For this review, take the finished solid that the model builds, in its own axes (mm). Face numbers are marked on the shaded views. Round coordinates to 2 decimals unless told otherwise and drop trailing zeros. Order: outer loops, then holes, each group sorted by start corner. A loop starts at its lowest first (then second) coordinate and runs counter-clockwise, first axis right, second up. Notation, with made-up numbers: M -26.5,3 L -17.5,3 A20 ccw -17.5,16 Z; hole C 74.25,8 d10. An arc over 180 degrees is marked long. Use a Markdown table: item, result.
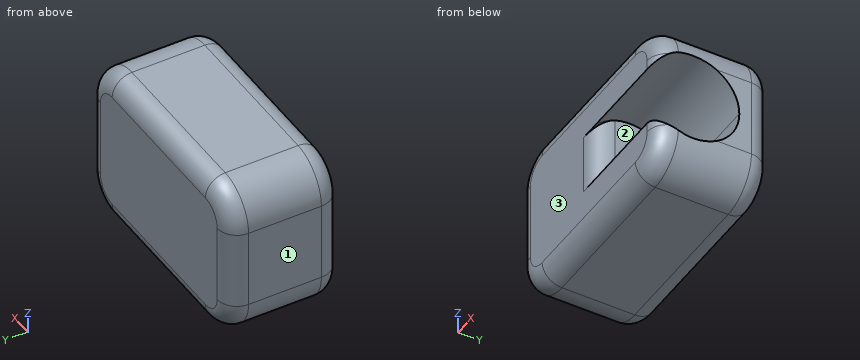
from build123d import *

# Parameters (mm, degrees)
F0_W         = 152.4
F0_H         = 101.6
F1_DEPTH     = 72.136
F3_DEPTH     = 69.088
F4_T1_DEPTH  = 199.136
F5_T1_DEPTH  = 101.6
F5_T3_DEPTH  = 50.8
F5_T5_DEPTH  = 37.8518945456
F5_T7_DEPTH  = 37.8518945456
F5_T12_DEPTH = 102.0962109088
F5_S13_R     = 29.4462721735
F5_T14_DEPTH = 53
F5_T16_ANGLE = 89.9999999994
F5_T18_ANGLE = 89.9999999994
F5_T20_ANGLE = 89.9999999994
F5_T22_ANGLE = 89.9999999994
F5_T24_ANGLE = 89.9999999994
F5_T26_ANGLE = 89.9999999994
F5_T28_ANGLE = 89.9999999994
F5_T30_ANGLE = 89.9999999994


# Not quite as in the source:
# - a fillet or chamfer that OpenCascade refuses, or shapes differently, is made with other operations: its cross-section is extruded or revolved along the edge and cut away or added


with BuildPart() as f1:
    # F0 (on Front) → F1 (new body)
    with BuildSketch(Plane.XZ):
        Rectangle(F0_W, F0_H)
    extrude(amount=F1_DEPTH)

    # F2 (on face) → F3 (cut)
    with BuildSketch(Plane.YZ.offset(76.2)):
        with BuildLine():
            Line((-72.136, -19.2981054544), (-72.136, 19.2981054544))
            ThreePointArc((-72.136, 19.2981054544), (-79.3411824793, 0), (-72.136, -19.2981054544))
        make_face()
        with BuildLine():
            ThreePointArc((-72.136, -19.2981054544), (-39.5952558372, -27.5862295855), (-20.4486381322, 0))
            ThreePointArc((-20.4486381322, 0), (-39.5952558372, 27.5862295855), (-72.136, 19.2981054544))
            Line((-72.136, 19.2981054544), (-72.136, -19.2981054544))
        make_face()
    extrude(amount=-F3_DEPTH, mode=Mode.SUBTRACT)

    # F4: fillet of radius 25.4 on 4 edges, made by hand

    # F4_s2 → F4_t1 (cut)
    with BuildSketch(Plane.XZ.offset(-63.5)):
        with BuildLine():
            ThreePointArc((50.8, -50.8), (68.7605122421, -43.3605122421), (76.2, -25.4))
            Line((76.2, -25.4), (76.2, -50.8))
            Line((76.2, -50.8), (50.8, -50.8))
        make_face()
        with BuildLine():
            ThreePointArc((-50.8, -50.8), (-68.7605122421, -43.3605122421), (-76.2, -25.4))
            Line((-76.2, -25.4), (-76.2, -50.8))
            Line((-76.2, -50.8), (-50.8, -50.8))
        make_face()
        with BuildLine():
            ThreePointArc((76.2, 25.4), (68.7605122421, 43.3605122421), (50.8, 50.8))
            Line((50.8, 50.8), (76.2, 50.8))
            Line((76.2, 50.8), (76.2, 25.4))
        make_face()
        with BuildLine():
            ThreePointArc((-76.2, 25.4), (-68.7605122421, 43.3605122421), (-50.8, 50.8))
            Line((-50.8, 50.8), (-76.2, 50.8))
            Line((-76.2, 50.8), (-76.2, 25.4))
        make_face()
    extrude(amount=F4_T1_DEPTH, mode=Mode.SUBTRACT)

    # F5: fillet of radius 12.7 on 16 edges, made by hand

    # F5_s2 → F5_t1 (cut)
    with BuildSketch(Plane.YZ.offset(-50.8)):
        with BuildLine():
            ThreePointArc((-72.136, 38.1), (-68.4162561211, 47.0802561211), (-59.436, 50.8))
            Line((-59.436, 50.8), (-72.136, 50.8))
            Line((-72.136, 50.8), (-72.136, 38.1))
        make_face()
        with BuildLine():
            ThreePointArc((0, 38.1), (-3.7197438789, 47.0802561211), (-12.7, 50.8))
            Line((-12.7, 50.8), (0, 50.8))
            Line((0, 50.8), (0, 38.1))
        make_face()
        with BuildLine():
            ThreePointArc((-12.7, -50.8), (-3.7197438789, -47.0802561211), (0, -38.1))
            Line((0, -38.1), (0, -50.8))
            Line((0, -50.8), (-12.7, -50.8))
        make_face()
        with BuildLine():
            ThreePointArc((-59.436, -50.8), (-68.4162561211, -47.0802561211), (-72.136, -38.1))
            Line((-72.136, -38.1), (-72.136, -50.8))
            Line((-72.136, -50.8), (-59.436, -50.8))
        make_face()
    extrude(amount=F5_T1_DEPTH, mode=Mode.SUBTRACT)

    # F5_s4 → F5_t3 (cut)
    with BuildSketch(Plane.XY.offset(-25.4)):
        with BuildLine():
            ThreePointArc((-63.5, 0), (-72.4802561211, -3.7197438789), (-76.2, -12.7))
            Line((-76.2, -12.7), (-76.2, 0))
            Line((-76.2, 0), (-63.5, 0))
        make_face()
        with BuildLine():
            ThreePointArc((63.5, 0), (72.4802561211, -3.7197438789), (76.2, -12.7))
            Line((76.2, -12.7), (76.2, 0))
            Line((76.2, 0), (63.5, 0))
        make_face()
        with BuildLine():
            ThreePointArc((-63.5, -72.136), (-72.4802561211, -68.4162561211), (-76.2, -59.436))
            Line((-76.2, -59.436), (-76.2, -72.136))
            Line((-76.2, -72.136), (-63.5, -72.136))
        make_face()
    extrude(amount=F5_T3_DEPTH, mode=Mode.SUBTRACT)

    # F5_s6 → F5_t5 (cut)
    with BuildSketch(Plane.XY.offset(-12.4518945456)):
        with BuildLine():
            ThreePointArc((63.5, -72.136), (72.4802561211, -68.4162561211), (76.2, -59.436))
            Line((76.2, -59.436), (76.2, -72.136))
            Line((76.2, -72.136), (63.5, -72.136))
        make_face()
    extrude(amount=F5_T5_DEPTH, mode=Mode.SUBTRACT)

    # F5_s8 → F5_t7 (cut)
    with BuildSketch(Plane.XY.offset(-25.4)):
        with BuildLine():
            ThreePointArc((63.5, -72.136), (72.4802561211, -68.4162561211), (76.2, -59.436))
            Line((76.2, -59.436), (76.2, -72.136))
            Line((76.2, -72.136), (63.5, -72.136))
        make_face()
    extrude(amount=F5_T7_DEPTH, mode=Mode.SUBTRACT)


with BuildPart() as f5_tool10:
    # F5_s11 → F5_t12 (new body)
    with BuildSketch(Plane.XY.offset(-51.0481054544)):
        with BuildLine():
            ThreePointArc((-5.588, -72.136), (3.3922561211, -68.4162561211), (7.112, -59.436))
            Line((7.112, -59.436), (7.112, -72.136))
            Line((7.112, -72.136), (-5.588, -72.136))
        make_face()
    extrude(amount=F5_T12_DEPTH)

    # F5_s13 → F5_t14 (intersect, symmetric)
    with BuildSketch(Plane.YZ.offset(0.8)):
        with Locations((-49.8949103057, 0)):
            Circle(F5_S13_R)
    extrude(amount=F5_T14_DEPTH, both=True, mode=Mode.INTERSECT)


with BuildPart() as f1_1:
    add(f1.part)

    # F5_t9: cut F5_tool10
    add(f5_tool10.part, mode=Mode.SUBTRACT)

    # F5_s15 → F5_t16 (revolve, cut)
    with BuildSketch(Plane.YZ.offset(-50.7999999999)):
        with BuildLine():
            ThreePointArc((0, -38.1), (-3.7197438789, -47.0802561211), (-12.7, -50.8))
            Line((-12.7, -50.8), (0, -50.8))
            Line((0, -50.8), (0, -38.1))
        make_face()
    revolve(axis=Axis((-50.7999999999, 0, -25.3999999999), (0, 1, 0)), revolution_arc=F5_T16_ANGLE, mode=Mode.SUBTRACT)

    # F5_s17 → F5_t18 (revolve, cut)
    with BuildSketch(Plane.XY.offset(25.3999999999)):
        with BuildLine():
            ThreePointArc((-63.5, 0), (-72.4802561211, -3.7197438789), (-76.2, -12.7))
            Line((-76.2, -12.7), (-76.2, 0))
            Line((-76.2, 0), (-63.5, 0))
        make_face()
    revolve(axis=Axis((-50.7999999999, 0, 25.3999999999), (0, 1, 0)), revolution_arc=F5_T18_ANGLE, mode=Mode.SUBTRACT)

    # F5_s19 → F5_t20 (revolve, cut)
    with BuildSketch(Plane.YZ.offset(50.7999999999)):
        with BuildLine():
            ThreePointArc((0, 38.1), (-3.7197438789, 47.0802561211), (-12.7, 50.8))
            Line((-12.7, 50.8), (0, 50.8))
            Line((0, 50.8), (0, 38.1))
        make_face()
    revolve(axis=Axis((50.7999999999, 0, 25.3999999999), (0, 1, 0)), revolution_arc=F5_T20_ANGLE, mode=Mode.SUBTRACT)

    # F5_s21 → F5_t22 (revolve, cut)
    with BuildSketch(Plane.XY.offset(-25.3999999999)):
        with BuildLine():
            ThreePointArc((63.5, 0), (72.4802561211, -3.7197438789), (76.2, -12.7))
            Line((76.2, -12.7), (76.2, 0))
            Line((76.2, 0), (63.5, 0))
        make_face()
    revolve(axis=Axis((50.7999999999, 0, -25.3999999999), (0, 1, 0)), revolution_arc=F5_T22_ANGLE, mode=Mode.SUBTRACT)

    # F5_s23 → F5_t24 (revolve, cut)
    with BuildSketch(Plane.XY.offset(-25.3999999999)):
        with BuildLine():
            ThreePointArc((76.2, -59.436), (72.4802561211, -68.4162561211), (63.5, -72.136))
            Line((63.5, -72.136), (76.2, -72.136))
            Line((76.2, -72.136), (76.2, -59.436))
        make_face()
    revolve(axis=Axis((50.7999999999, -72.136, -25.3999999999), (0, 1, 0)), revolution_arc=F5_T24_ANGLE, mode=Mode.SUBTRACT)

    # F5_s25 → F5_t26 (revolve, cut)
    with BuildSketch(Plane.XY.offset(25.3999999999)):
        with BuildLine():
            ThreePointArc((-63.5, -72.136), (-72.4802561211, -68.4162561211), (-76.2, -59.436))
            Line((-76.2, -59.436), (-76.2, -72.136))
            Line((-76.2, -72.136), (-63.5, -72.136))
        make_face()
    revolve(axis=Axis((-50.7999999999, -72.136, 25.3999999999), (0, 1, 0)), revolution_arc=F5_T26_ANGLE, mode=Mode.SUBTRACT)

    # F5_s27 → F5_t28 (revolve, cut)
    with BuildSketch(Plane.YZ.offset(50.7999999999)):
        with BuildLine():
            ThreePointArc((-72.136, 38.1), (-68.4162561211, 47.0802561211), (-59.436, 50.8))
            Line((-59.436, 50.8), (-72.136, 50.8))
            Line((-72.136, 50.8), (-72.136, 38.1))
        make_face()
    revolve(axis=Axis((50.7999999999, -72.136, 25.3999999999), (0, 1, 0)), revolution_arc=F5_T28_ANGLE, mode=Mode.SUBTRACT)

    # F5_s29 → F5_t30 (revolve, cut)
    with BuildSketch(Plane.YZ.offset(-50.7999999999)):
        with BuildLine():
            ThreePointArc((-72.136, -38.1), (-68.4162561211, -47.0802561211), (-59.436, -50.8))
            Line((-59.436, -50.8), (-72.136, -50.8))
            Line((-72.136, -50.8), (-72.136, -38.1))
        make_face()
    revolve(axis=Axis((-50.7999999999, -72.136, -25.3999999999), (0, 1, 0)), revolution_arc=F5_T30_ANGLE, mode=Mode.SUBTRACT)


solid = f1_1.part
Q1. Add section D-D (x = -9). Write out the cut boundary in (y, z), then the cut area to 3 significant figures.
Determined:
| item | result |
|---|---|
| outline | M -72.14,-38.1 A12.7 ccw -59.44,-50.8 L -12.7,-50.8 A12.7 ccw 0,-38.1 L 0,38.1 A12.7 ccw -12.7,50.8 L -59.44,50.8 A12.7 ccw -72.14,38.1 Z |
| area | 7,190 mm^2 |
Q2. Clearance check with flat-ended pins moving along their axes: pin 1 (3 mm diameter, centred on x = 55.5, y = -50.5, fed in from -Z); pin 2 (3 mm diameter, centred on y = -29.5, z = -37, fed in from +X); pin 3 (6 mm diameter, centred on y = -28.5, z = 31.5, fed in from +X). State where each tip first meets the part, or that it passes through.
Determined:
| item | result |
|---|---|
| pin 1 | stops at z = -50.6 |
| pin 2 | stops at x = 74.11 |
| pin 3 | stops at x = 76.01 |
Q3. Add section B-B (z = -8). Write out the cut boundary in (x, y).
Determined:
| item | result |
|---|---|
| outline | M -76.2,-59.44 A12.7 ccw -63.5,-72.14 L -5.59,-72.14 A12.7 ccw 7.11,-59.44 L 7.11,-21.56 L 76.2,-21.56 L 76.2,-12.7 A12.7 ccw 63.5,0 L -63.5,0 A12.7 ccw -76.2,-12.7 Z |
Q4. Wall thickness on line 1 along X through (y, z) = (-29.5, -25.5); line 2 along X through (y, z) = (-28, -4.5); line 3 along Z through (x, y) = (31, -33): over which ranges is each line inside the solid? List them lowest first. Write a range as [from, to].
Determined:
| item | result |
|---|---|
| line 1 | x = [-76.2, 76.2] |
| line 2 | x = [-76.2, 7.11] |
| line 3 | z = [-50.8, -24.12], [24.12, 50.8] |
Q5. Draft analysis for pull direction Y (two halves, no side actions). For the marked faces 1, 2 and 3, state which applies: pulls with the +Y half, pulls with the -Y half, needs draft (parallel to the pull), parting line crosses it, or undercut.
Determined:
| item | result |
|---|---|
| face 1 | needs draft |
| face 2 | undercut |
| face 3 | pulls with the -Y half |
Q6. Add section C-C (y = -51). Write out the cut boundary in (x, z), then the cut area to 3 significant figures.
Determined:
| item | result |
|---|---|
| outline | M -76.2,-25.4 A25.4 ccw -50.8,-50.8 L 50.8,-50.8 A25.4 ccw 75.88,-29.43 L 7.11,-29.43 L 7.11,29.43 L 75.88,29.43 A25.4 ccw 50.8,50.8 L -50.8,50.8 A25.4 ccw -76.2,25.4 Z |
| area | 10,900 mm^2 |
Q7. Add section A-A (x = 10.5). Write out the cut boundary in (y, z), then the cut area to 3 significant figures.
Determined:
| item | result |
|---|---|
| outline | M -72.14,-38.1 A12.7 ccw -59.44,-50.8 L -12.7,-50.8 A12.7 ccw 0,-38.1 L 0,38.1 A12.7 ccw -12.7,50.8 L -59.44,50.8 A12.7 ccw -72.14,38.1 L -72.14,19.3 A29.45 cw long -72.14,-19.3 Z |
| area | 4,660 mm^2 |
